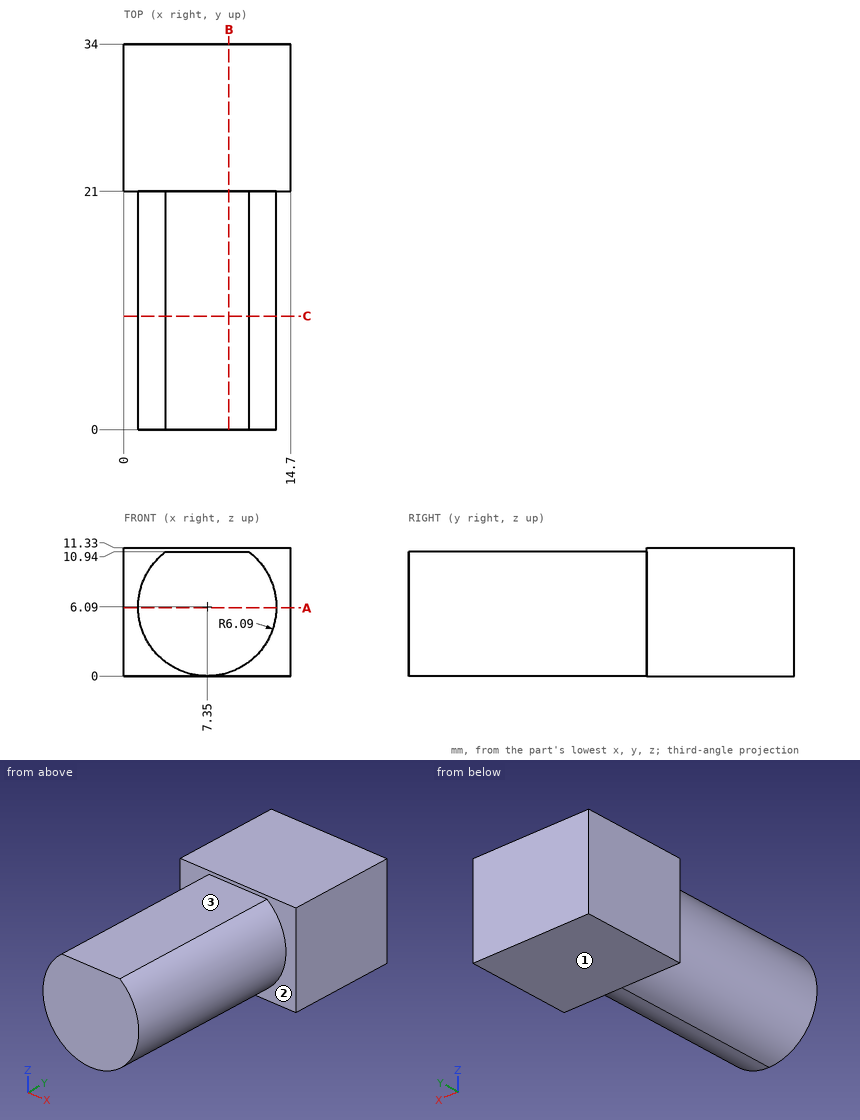
Input: dimensioned drawing with shaded views. Units: mm. Origin: part minimum x, y, z. A direction names the side the tool comes from. Coordinates: 2 decimals unless noted, no trailing zeros. Order: outer loops, then holes, each group sorted by start corner. A loop starts at its lowest first (then second) coordinate and runs counter-clockwise, first axis right, second up.
Item 1: Contact query for flat-ended pins moving along their axis: P1, Ø1.5, axis at y = 15, z = 10, coming from the +X side; P2, Ø1, axis at x = 10, y = 15, coming from the +Z side; P3, Ø1, axis at y = 10.5, z = 3, coming from the +X side. Output: stop coordinate, or through.
Answer:
P1: stops at x = 12.56
P2: stops at z = 10.94
P3: stops at x = 12.86
Item 2: Section query A-A (z = 6). Output: boundary loops of the cut face in (x, y), then the cut area to 3 significant figures.
Answer:
outline: (0, 21) - (1.26, 21) - (1.26, 0) - (13.44, 0) - (13.44, 21) - (14.7, 21) - (14.7, 34) - (0, 34) - close
area: 447 mm2
Item 3: Access query for the marked faces 1, 2 and 3. Directions: +Z, -Z, +X, -X, +Y, -Y. A direction counts if a zero-diameter tool reaches every point of the face in a straight line with its end or side. Return the directions, or none.
Answer:
face 1: -Z, +X, -X, +Y, -Y
face 2: -Y
face 3: +Z, +X, -X, -Y
Item 4: Section query B-B (x = 9.25). Output: boundary loops of the cut face in (y, z), then the cut area to 3 significant figures.
Answer:
outline: (0, 0.3) - (21, 0.3) - (21, 0) - (34, 0) - (34, 11.33) - (21, 11.33) - (21, 10.94) - (0, 10.94) - close
area: 371 mm2
Item 5: Section query C-C (y = 10). Output: boundary loops of the cut face in (x, z).
Answer:
outline: (3.67, 10.94) arc R6.09 ccw (long way) to (11.03, 10.94) - close
Item 6: Material intervals for line 1 along Y through (x, z) = (0.5, 5.5); line 2 along Z through (x, y) = (7.5, 3); line 3 along X through (y, z) = (2.5, 1), sorted ascending.
Answer:
line 1: y = 21 to 34
line 2: z = 0 to 10.94
line 3: x = 4.01 to 10.69
